Model file for the job. Use its own axes, mm. Coordinates: 2 decimals unless noted, no trailing zeros. Loops run counter-clockwise (first coordinate to the right, second up) from the corner with the lowest first, then second, coordinate; pieces in that order, holes last. Notation, with made-up numbers: (2.5, -5.5) -> (17.5, -5.5) arc R10 cw to (17.5, 4.5) -> close; hole circle Ø6 at (-12, -18). An arc over 180 degrees is marked (long way). Use one line per item in the form item = value.
```python
from build123d import *

# Parameters (mm, degrees)
SKETCH2_W           = 300
SKETCH2_H           = 300
BOSS_EXTRUDE1_DEPTH = 3
SKETCH3_R           = 15
CUT_EXTRUDE1_DEPTH  = 4
SKETCH4_R           = 5
CUT_EXTRUDE2_DEPTH  = 4


with BuildPart() as part:
    # Sketch2 → Boss-Extrude1 (new body)
    with BuildSketch(Plane(origin=(0, 0, 0), x_dir=(1, 0, 0), z_dir=(0, 1, 0))):
        Rectangle(SKETCH2_W, SKETCH2_H)
    extrude(amount=BOSS_EXTRUDE1_DEPTH)

    # Sketch3 → Cut-Extrude1 (cut, through all)
    with BuildSketch(Plane(origin=(0, 3, 0), x_dir=(1, 0, 0), z_dir=(0, 1, 0))):
        Circle(SKETCH3_R)
    extrude(amount=-CUT_EXTRUDE1_DEPTH, mode=Mode.SUBTRACT)

    # Sketch4 → Cut-Extrude2 (cut, through all)
    with BuildSketch(Plane(origin=(0, 3, 0), x_dir=(1, 0, 0), z_dir=(0, 1, 0))):
        with Locations((-120, 0)):
            Circle(SKETCH4_R)
    extrude(amount=-CUT_EXTRUDE2_DEPTH, mode=Mode.SUBTRACT)


solid = part.part
```
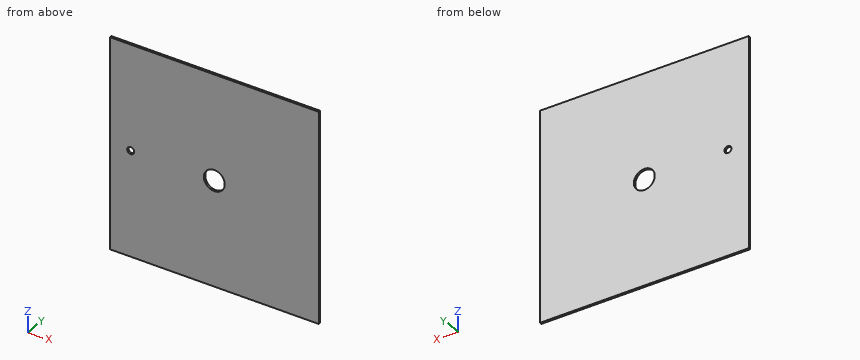
Q1. Band-saw the part on C-C, the plane x = 0. Write the cut outline in (y, z), and give its area (3 significant figures).
Result:
outline = (0, -150) -> (3, -150) -> (3, -15) -> (0, -15) -> close; (0, 15) -> (3, 15) -> (3, 150) -> (0, 150) -> close
area = 810 mm2
Q2. Wall check: line 1 along X through (y, z) = (0.9, 0); line 2 along Z through (x, y) = (-120, 2); line 3 along Z through (x, y) = (0, 2.4). Give the ranges that are in metal, low to high.
Result:
line_1 = -150 to -125, -115 to -15, 15 to 150
line_2 = -150 to -5, 5 to 150
line_3 = -150 to -15, 15 to 150
Q3. Band-saw the part on B-B, the plane x = -120. Write the cut outline in (y, z), and give its area (3 significant figures).
Result:
outline = (0, -150) -> (3, -150) -> (3, -5) -> (0, -5) -> close; (0, 5) -> (3, 5) -> (3, 150) -> (0, 150) -> close
area = 870 mm2
Q4. Band-saw the part on A-A, the plane z = 0. Write the cut outline in (x, y), and give its area (3 significant figures).
Result:
outline = (-150, 0) -> (-125, 0) -> (-125, 3) -> (-150, 3) -> close; (-115, 0) -> (-15, 0) -> (-15, 3) -> (-115, 3) -> close; (15, 0) -> (150, 0) -> (150, 3) -> (15, 3) -> close
area = 780 mm2
